Verification items for the finished model (mm, model axes). A direction names the side the tool comes from. Round coordinates to 2 decimals unless told otherwise and drop trailing zeros. Put each result on its own line as item: value.
from build123d import *

# Parameters (mm, degrees)
BOSS_EXTRUDE1_DEPTH     = 7.5
CUT_EXTRUDE1_DEPTH      = 4
FILLET1_R               = 10
CUT_EXTRUDE_THIN2_START = -0.5
SKETCH2_W               = 1
SKETCH2_H               = 80
CUT_EXTRUDE_THIN2_DEPTH = 71.201147767
CIRPATTERN1_COUNT       = 13
CIRPATTERN1_ANGLE       = 90
SKETCH5_R               = 2
CUT_EXTRUDE2_DEPTH      = 2


with BuildPart() as part:
    # Sketch1 → Boss-Extrude1 (new body)
    with BuildSketch(Plane(origin=(0, 0, 0), x_dir=(0, 1, 0), z_dir=(0, 0, 1))):
        Polygon((44, 49), (49, 44), (49, 0), (0, 0), (0, 49), align=None)
    extrude(amount=BOSS_EXTRUDE1_DEPTH)

    # Sketch4 → Cut-Extrude1 (cut)
    with BuildSketch(Plane.XY.offset(7.5)):
        with BuildLine():
            Line((-48, 33.585786438), (-48, 43.585786438))
            Line((-48, 43.585786438), (-43.585786438, 48))
            Line((-43.585786438, 48), (-33.585786438, 48))
            ThreePointArc((-33.585786438, 48), (-37.679974138, 37.679974138), (-48, 33.585786438))
        make_face()
    extrude(amount=-CUT_EXTRUDE1_DEPTH, mode=Mode.SUBTRACT)

    # Fillet1
    # the kernel refuses this fillet: 10 mm, written as the material it adds along each edge
    with BuildSketch(Plane(origin=(-47.579469074, 47.579469074, 3.5), x_dir=(0.11133254598892352, 0.9937832078494908, 0), z_dir=(-0.9937832078494908, 0.11133254598892352, 0))) as fillet1_piece_1_section:
        with BuildLine():
            CenterArc((6, -10), FILLET1_R, 36.869897646, 53.130102354)
            Line((6, 0), (6, 0.2))
            Line((6, 0.2), (14, 0.2))
            Line((14, 0.2), (14.2, 0))
            ThreePointArc((14.2, 0), (14.2, -2), (14.16, -3.88))
            Line((14.16, -3.88), (14, -4))
        make_face()
    fillet1_piece_1 = revolve(axis=Axis((-47.579469074, 47.579469074, 3.5), (0, 0, -1)), revolution_arc=257.215726598, mode=Mode.PRIVATE)
    fillet1_piece_1 = split(fillet1_piece_1, bisect_by=Plane(origin=(-48, 39.87908293, 4.608055209), z_dir=(1, 0, 0)), keep=Keep.TOP, mode=Mode.PRIVATE)
    fillet1_piece_1 = split(fillet1_piece_1, bisect_by=Plane(origin=(-39.879083288, 48, 4.608055209), z_dir=(0, -1, 0)), keep=Keep.TOP, mode=Mode.PRIVATE)
    add(fillet1_piece_1)

    # Sketch2 → Cut-Extrude-Thin2 (cut)
    with BuildSketch(Plane.XY.offset(7.5).offset(CUT_EXTRUDE_THIN2_START)):
        with Locations((-46.5, 4.585786438)):
            Rectangle(SKETCH2_W, SKETCH2_H)
    cut_extrude_thin2 = extrude(amount=CUT_EXTRUDE_THIN2_DEPTH, mode=Mode.SUBTRACT)

    # CirPattern1: Cut-Extrude-Thin2 ×13 about axis
    cirpattern1_axis = Axis((-46.5, 46.5, 0), (0, 0, 1))
    for i in range(1, CIRPATTERN1_COUNT):
        add(cut_extrude_thin2.rotate(cirpattern1_axis, i * CIRPATTERN1_ANGLE / (CIRPATTERN1_COUNT - 1)), mode=Mode.SUBTRACT)

    # Sketch5 → Cut-Extrude2 (cut)
    with BuildSketch(Plane(origin=(0, 0, 0), x_dir=(0, 1, 0), z_dir=(0, 0, 1))):
        with Locations(Location((24.5, 26.5, 0), (0, 0, 270))):
            Circle(SKETCH5_R)
    extrude(amount=CUT_EXTRUDE2_DEPTH, mode=Mode.SUBTRACT)


solid = part.part
Item 1: Gauge pin test, flat ends, axial feed: pin 1 Ø2 at (x, y) = (-26.5, 24) entering from -Z; pin 2 Ø2 at (x, z) = (-41, 4.5) entering from -Y; pin 3 Ø0.8 at (x, y) = (-46.5, 11) entering from +Z. Record the tip position at first contact, or that the pin passes through.
Check sheet entries:
pin 1: stops at z = 2
pin 2: stops at y = 0
pin 3: stops at z = 7
Item 2: Tool access check on faces 1 (the flat face through (-40, 13, 7.5)), 2 (the flat face through (-48, 40, 6)), 3 (the cylindrical face through (-25.577, 22.726, 0.986)). Record the directions out of +Z, -Z, +X, -X, +Y, -Y that give a thin tool (end or side, any length) a straight path to the whole face; none if there is none.
Check sheet entries:
face 1: +Z, +X, -X, +Y, -Y
face 2: +Z
face 3: -Z
Item 3: Material ranges on L1, parallel to Y at x = -26.5, z = 1.3; L2, parallel to Y at x = -26, z = 0.5; L3, parallel to Z at x = -25.5, y = 30.5, recorded low to high. Write a range as [from, to].
Check sheet entries:
L1: y = [0, 22.5], [26.5, 49]
L2: y = [0, 22.56], [26.44, 49]
L3: z = [0, 7]
Item 4: Release check for a two-part mould opening along X. For faces 4 (the flat face through (-18, 39, 7)), 5 (the flat face through (-35, 12, 7.5)), 6 (the flat face through (-49, 22, 4)) record: +X half, -X half, draft (parallel to the pull), parting line (faces both ways), or undercut.
Check sheet entries:
face 4: undercut
face 5: draft
face 6: -X half
